```python
from build123d import *

# Parameters (mm, degrees)
F0_R     = 38
F0_W     = 3
F0_H     = 2
F1_DEPTH = 2


with BuildPart() as f1:
    # F0 (on Right) → F1 (new body)
    with BuildSketch(Plane.YZ):
        with BuildLine():
            Line((-146.682539, 58.671261), (-146.682539, 55.671261))
            Line((-146.682539, 55.671261), (-146.682539, 53.671261))
            Line((-146.682539, 53.671261), (-146.682539, 51.671261))
            Line((-146.682539, 51.671261), (-171.682539, 51.671261))
            Line((-171.682539, 51.671261), (-171.682539, -9.328739))
            ThreePointArc((-171.682539, -9.328739), (-167.289141, -19.935341), (-156.682539, -24.328739))
            Line((-156.682539, -24.328739), (-56.206871, -24.328739))
            Line((-56.206871, -24.328739), (35.424741, -24.216021))
            ThreePointArc((35.424741, -24.216021), (42.4922, -21.278392), (45.412432, -14.203727))
            Line((45.412432, -14.203727), (45.407673, -10.334779))
            ThreePointArc((45.407673, -10.334779), (47.586471, -4.091191), (53.185443, -0.572517))
            Line((53.185443, -0.572517), (74.875972, 4.371213))
            Line((74.875972, 4.371213), (89.500913, 7.704547))
            Line((89.500913, 7.704547), (89.034246, 9.752038))
            Line((89.034246, 9.752038), (103.659187, 13.085372))
            Line((103.659187, 13.085372), (104.125853, 11.03788))
            Line((104.125853, 11.03788), (118.750794, 14.371213))
            Line((118.750794, 14.371213), (129.528572, 16.827697))
            ThreePointArc((129.528572, 16.827697), (132.32614, 18.584629), (133.417461, 21.702677))
            Line((133.417461, 21.702677), (133.417461, 51.671261))
            Line((133.417461, 51.671261), (118.317461, 51.671261))
            Line((118.317461, 51.671261), (118.317461, 53.671261))
            Line((118.317461, 53.671261), (118.317461, 55.671261))
            Line((118.317461, 55.671261), (118.317461, 58.671261))
            ThreePointArc((118.317461, 58.671261), (116.852995, 62.206795), (113.317461, 63.671261))
            Line((113.317461, 63.671261), (-141.682539, 63.671261))
            ThreePointArc((-141.682539, 63.671261), (-145.218073, 62.206795), (-146.682539, 58.671261))
        make_face()
        Polygon((-123.432658, -7.662072), (-138.057599, -10.995406), (-138.524265, -8.947914), (-123.899325, -5.614581), align=None, mode=Mode.SUBTRACT)
        Polygon((-155.079492, 5.637848), (-157.126984, 5.171182), (-160.460317, 19.796122), (-158.412825, 20.262789), align=None, mode=Mode.SUBTRACT)
        Polygon((-116.585495, 29.796122), (-113.252162, 15.171182), (-115.299654, 14.704515), (-118.632987, 29.329456), align=None, mode=Mode.SUBTRACT)
        with Locations((-61.929516, 20.671261)):
            Circle(F0_R, mode=Mode.SUBTRACT)
        Polygon((72.479019, 24.337801), (70.431528, 23.871134), (67.098194, 38.496075), (69.145686, 38.962742), align=None, mode=Mode.SUBTRACT)
        Polygon((110.973016, 48.496075), (114.30635, 33.871134), (112.258858, 33.404468), (108.925524, 48.029408), align=None, mode=Mode.SUBTRACT)
        with Locations((119.817461, 54.671261)):
            Rectangle(F0_W, F0_H)
        with Locations((-148.182539, 54.671261)):
            Rectangle(F0_W, F0_H)
    extrude(amount=F1_DEPTH)


solid = f1.part
```
Build history of the part. All positions in model axes, mm. Give positions to 0.01 mm unless a question says otherwise; leave off trailing zeros. Order: outer loops, then holes, each group sorted by start corner. A loop starts at its lowest first (then second) coordinate and runs counter-clockwise, first axis right, second up. Notation, with made-up numbers: M 9,85.25 L 66,85.25 A22 cw 66,93.25 Z; hole C -31.5,4.5 d5. An arc over 180 degrees is marked long. Write item = value, one per line. Start each with the question number.
(1) Slice it at A-A on y = -81.5. Write the cut outline in (x, z), plus the area to 3 significant figures.
(2) Two-plate mould, pull along Z, no slides. Class faces 1 (the cylindrical face through (0.986, -25.684, 32.085)), 2 (the cylindrical face through (0.99, 116.89, 62.17)), 3 (the flat face through (2, -21, 20)): released by +Z, released by -Z, zero draft, split by the parting line, or undercut.
(3) Pin check, flat tips, straight feed: pin 1 Ø1 at (x, z) = (1, 55) entering from -Y; pin 2 Ø0.6 at (x, y) = (1, 124) entering from +Z. Stop position of each tip, or through.
(4) Probe L1, parallel to Y at x = 1.3, z = 19.5; L2, parallel to Y at x = 0.85, z = 28.5; L3, parallel to Y at x = 1.35, z = 21.5. List the from-to ranges inside material, lowest first. Write a range as [from, to].
(5) Slice it at B-B on x = 0.9. State how many separate pieces and enclosed holes the cut face has, plus the area to 3 significant figures.
Responses:
q1.outline = M 0,-24.33 L 2,-24.33 L 2,-11.9 L 0,-11.9 Z; M 0,53.24 L 2,53.24 L 2,63.67 L 0,63.67 Z
q1.area = 45.7 mm2
q2.face_1 = undercut
q2.face_2 = released by +Z
q2.face_3 = zero draft
q3.pin_1 = -149.68
q3.pin_2 = 51.67
q4.L1 = [-171.68, -160.39], [-158.24, -116.39], [-114.24, -99.91], [-23.95, 132.91]
q4.L2 = [-171.68, -118.44], [-116.29, -99.11], [-24.74, 69.38], [71.53, 133.42]
q4.L3 = [-171.68, -116.85], [-114.69, -99.92], [-23.94, 133.41]
q5.separate_pieces = 1
q5.enclosed_holes = 6
q5.area = 18,800 mm2
